from build123d import *

# Parameters (mm, degrees)
ESQUISSE1_W        = 19
ESQUISSE1_H        = 63
ESQUISSE1_R        = 1
BOSS_EXTRU_1_DEPTH = 1.5
BOSS_EXTRU_2_DEPTH = 2


with BuildPart() as part:
    # Esquisse1 → Boss.-Extru.1 (new body)
    with BuildSketch(Plane.XY):
        Rectangle(ESQUISSE1_W, ESQUISSE1_H)
        with Locations((-7, 29.5)):
            Circle(ESQUISSE1_R, mode=Mode.SUBTRACT)
        with Locations(Location((7, 29.5, 0), (0, 0, 180))):
            Circle(ESQUISSE1_R, mode=Mode.SUBTRACT)
    extrude(amount=BOSS_EXTRU_1_DEPTH)

    # Esquisse2 → Boss.-Extru.2 (add)
    with BuildSketch(Plane(origin=(0, 0, 0), x_dir=(-1, 0, 0), z_dir=(0, 0, -1))):
        with BuildLine():
            Line((-4, 31.5), (-4, 27.5))
            ThreePointArc((-4, 27.5), (-3.707106781, 26.792893219), (-3, 26.5))
            Line((-3, 26.5), (3, 26.5))
            ThreePointArc((3, 26.5), (3.707106781, 26.792893219), (4, 27.5))
            Line((4, 27.5), (4, 31.5))
            Line((4, 31.5), (-4, 31.5))
        make_face()
    extrude(amount=BOSS_EXTRU_2_DEPTH)


solid = part.part
Could you check a few things on this model? Use its own coordinates, in mm. A direction names the side the tool comes from. Give positions to 0.01 mm unless a question says otherwise; leave off trailing zeros. Write each loop counter-clockwise with the first axis right and the second up, starting at its lowest first coordinate (ties: lowest second). Pieces come first, ordered by that corner, then holes. Notation, with made-up numbers: (-18, -34) - (-12, -34) arc R23 ccw to (-12, -9) - close; hole circle Ø7 at (74, 65.25). An arc over 180 degrees is marked (long way). Use CSV: the item, a comma, the result in double quotes. Start each with the question number.
Item 1: For faces 5 (the face through (0, 26.5, -1)), 6 (the face through (3.715, 26.801, -0.986)), 7 (the face through (4, 30, -1)), which set-ups out of +Z, -Z, +X, -X, +Y, -Y let a thin tool reach every point of the face, with its end or its side?
Item 2: I want a section at A-A, the plane x = 7. Please give me the cut outline in (y, z).
Item 3: I want a section at C-C, the plane x = 2.25. Please give me the cut outline in (y, z).
Item 4: I want a section at B-B, the plane y = 29.5. Please give me the cut outline in (x, z).
Item 5: If we mould it in two halves opening along Y, with no side actions, what happens to faces 1 (the face through (7.13, 28.51, 0.74)), 2 (the face through (0, -31.5, 1)), 3 (the face through (-7.13, 30.49, 0.74)), 4 (the face through (-4, 29, -1))? For each: pulls with the +Y half, pulls with the -Y half, needs draft (parallel to the pull), parting line crosses it, or undercut.
Item 6: I'm going to push flat-ended pins straight in: pin 1 (2 mm diameter, centred on y = 30.5, z = -1.5, fed in from +X); pin 2 (1.6 mm diameter, centred on x = 1, z = -1, fed in from -Y); pin 3 (10 mm diameter, centred on x = 3.5, y = -12.5, fed in from -Z); pin 4 (1.6 mm diameter, centred on x = -7, y = 29.5, fed in from +Z). Where does each tip first touch, or does it pass through?
Item 7: I want a section at D-D, the plane y = -8. Please give me the cut outline in (x, z).
Item 8: If I drill on line 1 along Y through (x, z) = (7, 0.45); line 2 along Z through (x, y) = (-6.25, 4.5); line 3 along Y through (x, z) = (0.75, -0.2), over which ranges is the centre line in solid material (lowest first)?
Findings:
1,face 5,"-Z, +X, -X, -Y"
1,face 6,"-Z, +X, -Y"
1,face 7,"-Z, +X, +Y, -Y"
2,outline,"(-31.5, 0) - (28.5, 0) - (28.5, 1.5) - (-31.5, 1.5) - close; (30.5, 0) - (31.5, 0) - (31.5, 1.5) - (30.5, 1.5) - close"
3,outline,"(-31.5, 0) - (26.5, 0) - (26.5, -2) - (31.5, -2) - (31.5, 1.5) - (-31.5, 1.5) - close"
4,outline,"(-9.5, 0) - (-8, 0) - (-8, 1.5) - (-9.5, 1.5) - close; (-6, 0) - (-4, 0) - (-4, -2) - (4, -2) - (4, 0) - (6, 0) - (6, 1.5) - (-6, 1.5) - close; (8, 0) - (9.5, 0) - (9.5, 1.5) - (8, 1.5) - close"
5,face 1,"undercut"
5,face 2,"pulls with the -Y half"
5,face 3,"undercut"
5,face 4,"needs draft"
6,pin 1,"stops at x = 4"
6,pin 2,"stops at y = 26.5"
6,pin 3,"stops at z = 0"
6,pin 4,"passes through"
7,outline,"(-9.5, 0) - (9.5, 0) - (9.5, 1.5) - (-9.5, 1.5) - close"
8,line 1,"y = -31.5 to 28.5, 30.5 to 31.5"
8,line 2,"z = 0 to 1.5"
8,line 3,"y = 26.5 to 31.5"
